Verification items for the finished model (mm, model axes). Face numbers are marked on the shaded views. A direction names the side the tool comes from. Give positions to 0.01 mm unless a question says otherwise; leave off trailing zeros. Order: outer loops, then holes, each group sorted by start corner. A loop starts at its lowest first (then second) coordinate and runs counter-clockwise, first axis right, second up. Notation, with made-up numbers: M 62.25,52 L 99.25,52 A21 cw 99.25,66 Z; hole C 1,57.5 d10. An arc over 180 degrees is marked long. Answer as a JSON object with one key per item and string values.
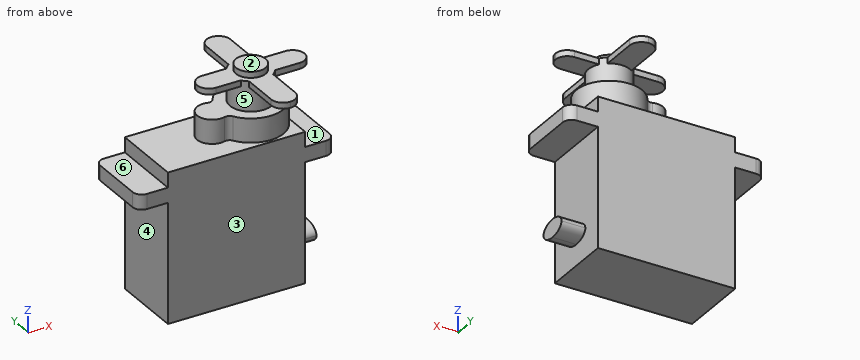
Autodesk Fusion 360 part; units mm, degrees
sketch "Skizze1" plane through (0, 0, 0) normal (0, 0, 1) x (1, 0, 0)
  line L0 (11.5, 6) -> (-11.5, 6)
  line L1 (-11.5, 6) -> (-11.5, -6)
  line L2 (-11.5, -6) -> (11.5, -6)
  line L3 (11.5, -6) -> (11.5, 6)
  line L4 (11.5, 6) -> (-11.5, -6) construction
  line L5 (-11.5, 6) -> (11.5, -6) construction
  dimension "d1" = 23
  dimension "d2" = 12
extrude "Extrusion1" add sketch "Skizze1" along normal mid plane 25
sketch "Skizze2" plane through (0, -6, 0) normal (0, -1, 0) x (1, 0, 0)
  line L0 (11.5, -12.5) -> (11.5, 12.5)
  line L1 (11.5, 12.5) -> (-11.5, 12.5)
  line L2 (-11.5, 12.5) -> (-11.5, -12.5)
  line L3 (-11.5, -12.5) -> (11.5, -12.5)
  line L4 (-16.5, 10) -> (16.5, 10)
  line L5 (16.5, 10) -> (16.5, 7.5)
  line L6 (16.5, 7.5) -> (-16.5, 7.5)
  line L7 (-16.5, 7.5) -> (-16.5, 10)
  dimension "d5" = 2.5
  dimension "d6" = 2.5
  dimension "d7" = 5
  dimension "d8" = 5
extrude "Extrusion2" add sketch "Skizze2" against normal blind 12 contours L0 L4 L5 L6 | L2 L4 L6 L7
fillet "Abrundung1" radius 1.5 4 edges at (16.5, -6, 8.75) (16.5, 6, 8.75) (-16.5, -6, 8.75) (-16.5, 6, 8.75)
sketch "Skizze3" plane through (0, 0, 12.5) normal (0, 0, 1) x (1, 0, 0)
  line L0 (11.5, -6) -> (11.5, 6)
  line L1 (11.5, 6) -> (-11.5, 6)
  line L2 (-11.5, 6) -> (-11.5, -6)
  line L3 (-11.5, -6) -> (11.5, -6)
  circle A0 centre (6, 0) radius 5.5
  circle A1 centre (-0.5, 0) radius 2.5
  dimension "d13" = 11
  dimension "d15" = 5
  dimension "d16" = 12
extrude "Extrusion3" add sketch "Skizze3" along normal blind 4 contours A0 A1 | A0 A1 | A0 A1
fillet "Abrundung2" radius 1 2 edges at (0.9038, -2.0686, 14.5) (0.9038, 2.0686, 14.5)
sketch "Skizze4" plane through (11.5, 0, 0) normal (1, 0, 0) x (0, 0, -1)
  line L0 (-7.5, 6) -> (-7.5, -6)
  line L1 (-7.5, -6) -> (12.5, -6)
  line L2 (12.5, -6) -> (12.5, 6)
  line L3 (12.5, 6) -> (-7.5, 6)
  ellipse E0 centre (7.5, 0) end of major axis (7.5, 2.5) minor radius 1.5
  line L4 (7.5, -2.5) -> (7.5, 2.5)
  line L5 (9, 0) -> (6, 0)
  dimension "d21" = 5
  dimension "d22" = 3
  dimension "d23" = 5
extrude "Extrusion4" add sketch "Skizze4" along normal blind 4 contours E0 L4 L5 | E0 L4 L5 | E0 L4 L5 | E0 L4 L5
sketch "Skizze5" plane through (0, 0, 16.5) normal (0, 0, 1) x (1, 0, 0)
  arc A0 (1.2973, -2.8522) -> (1.2973, 2.8522) centre (6, 0) ccw
  arc A1 (0.1731, 2.4077) -> (1.2973, 2.8522) centre (0.4423, 3.3708) ccw
  arc A2 (0.1731, 2.4077) -> (0.1731, -2.4077) centre (-0.5, 0) ccw
  arc A3 (1.2973, -2.8522) -> (0.1731, -2.4077) centre (0.4423, -3.3708) ccw
  circle A4 centre (6, 0) radius 3.5
  dimension "d26" = 7
extrude "Extrusion5" add sketch "Skizze5" along normal blind 4 contours A4
sketch "Skizze6" plane through (0, 0, 20.5) normal (0, 0, 1) x (1, 0, 0)
  circle A0 centre (6, 0) radius 3.5
  line L0 (8, 11) -> (4, 11)
  line L1 (4, -11) -> (8, -11)
  line L2 (8, 11) -> (4, -11) construction
  line L3 (4, 11) -> (8, -11) construction
  line L4 (-3, -2) -> (-3, 2)
  line L5 (15, 2) -> (15, -2)
  line L6 (15, -2) -> (-3, 2) construction
  line L7 (-3, -2) -> (15, 2) construction
  line L8 (-3, 2) -> (3.1277, 2)
  line L9 (5.6364, 2) -> (6.3636, 2)
  line L10 (8.8723, 2) -> (15, 2)
  line L11 (4, 11) -> (4, 2.8723)
  line L12 (8, 2.8723) -> (8, 11)
  line L13 (8, -11) -> (8, -2)
  line L14 (8, -0.4444) -> (8, 0.4444)
  line L15 (15, -2) -> (8.8723, -2)
  line L16 (6.3636, -2) -> (5.6364, -2)
  line L17 (3.1277, -2) -> (-3, -2)
  line L18 (4, 0.4444) -> (4, -0.4444)
  line L19 (4, -2.8723) -> (4, -11)
  point P0 (6, 0)
  point P1 (6, 0)
  dimension "d29" = 4
  dimension "d30" = 4
  dimension "d31" = 18
  dimension "d32" = 22
extrude "Extrusion6" add sketch "Skizze6" along normal blind 1
fillet "Abrundung3" radius 2 8 edges at (-3, -2, 21) (4, -11, 21) (8, -11, 21) (15, -2, 21) (15, 2, 21) (8, 11, 21) (4, 11, 21) (-3, 2, 21)
sketch "Skizze7" plane through (0, 0, 21.5) normal (0, 0, 1) x (1, 0, 0)
  arc A0 (-1, 2) -> (-1, -2) centre (-1, 0) ccw
  line L0 (-1, -2) -> (3.1277, -2)
  arc A1 (3.1277, -2) -> (4, -2.8723) centre (6, 0) ccw
  line L1 (4, -2.8723) -> (4, -9)
  arc A2 (4, -9) -> (8, -9) centre (6, -9) ccw
  line L2 (8, -9) -> (8, -2.8723)
  arc A3 (8, -2.8723) -> (8.8723, -2) centre (6, 0) ccw
  line L3 (8.8723, -2) -> (13, -2)
  arc A4 (13, -2) -> (13, 2) centre (13, 0) ccw
  line L4 (13, 2) -> (8.8723, 2)
  arc A5 (8.8723, 2) -> (8, 2.8723) centre (6, 0) ccw
  line L5 (8, 2.8723) -> (8, 9)
  arc A6 (8, 9) -> (4, 9) centre (6, 9) ccw
  line L6 (4, 9) -> (4, 2.8723)
  arc A7 (4, 2.8723) -> (3.1277, 2) centre (6, 0) ccw
  line L7 (3.1277, 2) -> (-1, 2)
  circle A8 centre (6, 0) radius 2.5
  dimension "d37" = 5
extrude "Extrusion7" add sketch "Skizze7" along normal blind 1 contours A8
equation "d8 = d7"
equation "d30 = d29"
Q1. Section check A-A on x = -0.5. Record the cut outline in (y, z), then the cut area to 3 significant figures.
Resolved:
{"outline": "M -6,-12.5 L 6,-12.5 L 6,12.5 L 2.5,12.5 L 2.5,16.5 L -2.5,16.5 L -2.5,12.5 L -6,12.5 Z; M -2,20.5 L 2,20.5 L 2,21.5 L -2,21.5 Z", "area": "324 mm²"}
Q2. Gauge pin test, flat ends, axial feed: pin 1 Ø3.5 at (x, y) = (4, -2.5) entering from +Z; pin 2 Ø4 at (x, y) = (-14.5, -1.5) entering from -Z; pin 3 Ø12.5 at (x, z) = (1.5, 0.5) entering from -Y; pin 4 Ø1.5 at (x, y) = (13, 1) entering from +Z. Record the tip position at first contact, or that the pin passes through.
Resolved:
{"pin 1": "stops at z = 22.5", "pin 2": "stops at z = 7.5", "pin 3": "stops at y = -6", "pin 4": "stops at z = 21.5"}
Q3. Release check for a two-part mould opening along Z. For the marked faces 1, 2 and 3 record: +Z half, -Z half, draft (parallel to the pull), parting line (faces both ways), or undercut.
Resolved:
{"face 1": "undercut", "face 2": "+Z half", "face 3": "draft"}
Q4. Material ranges on L1, parallel to Z at x = 5, y = 4.5; L2, parallel to Y at x = -2, z = 3; L3, parallel to Z at x = -3, y = 5.25, recorded low to high.
Resolved:
{"L1": "z = -12.5 to 16.5, 20.5 to 21.5", "L2": "y = -6 to 6", "L3": "z = -12.5 to 12.5"}
Q5. Tool access check on the marked faces 4, 5 and 6. Record the directions out of +Z, -Z, +X, -X, +Y, -Y that give a thin tool (end or side, any length) a straight path to the whole face; none if there is none.
Resolved:
{"face 4": "-Z, -X, +Y, -Y", "face 5": "none", "face 6": "+Z, -X, +Y, -Y"}
Q6. Section check B-B on x = -10. Record the cut outline in (y, z).
Resolved:
{"outline": "M -6,-12.5 L 6,-12.5 L 6,12.5 L -6,12.5 Z"}
Q7. Section check C-C on z = -3. Record the cut outline in (x, y).
Resolved:
{"outline": "M -11.5,-6 L 11.5,-6 L 11.5,6 L -11.5,6 Z"}
